Read the model definition and answer for the solid it produces. Units are mm, in the model's axes. Give positions to 0.01 mm unless a question says otherwise; leave off trailing zeros. Write each question's results on one line, items separated by ' | '.
from build123d import *

# Parameters (mm, degrees)
BOSS_EXTRUDE1_DEPTH  = 600
MIRROR3_COPY_1_DEPTH = 600
MIRROR3_COPY_2_DEPTH = 600


with BuildPart() as part:
    # Sketch1 → Boss-Extrude1 (new body)
    with BuildSketch(Plane.XY):
        with BuildLine():
            Line((3.4, 0), (5.5, 0))
            Line((5.5, 0), (5.5, 4))
            Line((5.5, 4), (11.69, 10.19))
            Line((11.69, 10.19), (18.2, 10.19))
            Line((18.2, 10.19), (18.2, 5.265595036))
            Line((18.2, 5.265595036), (15.5, 5.265595036))
            Line((15.5, 5.265595036), (15.5, 2.965595036))
            Line((15.5, 2.965595036), (19, 2.965595036))
            Line((19, 2.965595036), (19, 3.965595036))
            Line((19, 3.965595036), (20, 3.965595036))
            Line((20, 3.965595036), (20, 15.5))
            ThreePointArc((20, 15.5), (18.681980515, 18.681980515), (15.5, 20))
            Line((15.5, 20), (6.385304712, 20))
            Line((6.385304712, 20), (6.385304712, 19))
            Line((6.385304712, 19), (5.385304712, 19))
            Line((5.385304712, 19), (5.385304712, 15.5))
            Line((5.385304712, 15.5), (7.685304712, 15.5))
            Line((7.685304712, 15.5), (7.685304712, 18.2))
            Line((7.685304712, 18.2), (10.19, 18.2))
            Line((10.19, 18.2), (10.19, 11.69))
            Line((10.19, 11.69), (4, 5.5))
            Line((4, 5.5), (0, 5.5))
            Line((0, 5.5), (0, 3.4))
            ThreePointArc((0, 3.4), (2.404163056, 2.404163056), (3.4, 0))
        make_face()
        with BuildLine():
            Line((18.5, 11.69), (18.5, 15.5))
            ThreePointArc((18.5, 15.5), (17.621320344, 17.621320344), (15.5, 18.5))
            Line((15.5, 18.5), (11.69, 18.5))
            Line((11.69, 18.5), (11.69, 11.69))
            Line((11.69, 11.69), (18.5, 11.69))
        make_face(mode=Mode.SUBTRACT)
    boss_extrude1 = extrude(amount=BOSS_EXTRUDE1_DEPTH)

    # Mirror1: Boss-Extrude1 across plane
    add(boss_extrude1.mirror(Plane.ZX))

    # Mirror2: Boss-Extrude1 across plane
    add(boss_extrude1.mirror(Plane(origin=(0, 0, 0), x_dir=(0, 0, 1), z_dir=(1, 0, 0))))

    # Mirror3 copy 1 sketch → Mirror3 copy 1 (add)
    with BuildSketch(Plane(origin=(0, 0, 0), x_dir=(-1, 0, 0), z_dir=(0, 0, 1))):
        with BuildLine():
            Line((3.4, 0), (5.5, 0))
            Line((5.5, 0), (5.5, 4))
            Line((5.5, 4), (11.69, 10.19))
            Line((11.69, 10.19), (18.2, 10.19))
            Line((18.2, 10.19), (18.2, 5.265595036))
            Line((18.2, 5.265595036), (15.5, 5.265595036))
            Line((15.5, 5.265595036), (15.5, 2.965595036))
            Line((15.5, 2.965595036), (19, 2.965595036))
            Line((19, 2.965595036), (19, 3.965595036))
            Line((19, 3.965595036), (20, 3.965595036))
            Line((20, 3.965595036), (20, 15.5))
            ThreePointArc((20, 15.5), (18.681980515, 18.681980515), (15.5, 20))
            Line((15.5, 20), (6.385304712, 20))
            Line((6.385304712, 20), (6.385304712, 19))
            Line((6.385304712, 19), (5.385304712, 19))
            Line((5.385304712, 19), (5.385304712, 15.5))
            Line((5.385304712, 15.5), (7.685304712, 15.5))
            Line((7.685304712, 15.5), (7.685304712, 18.2))
            Line((7.685304712, 18.2), (10.19, 18.2))
            Line((10.19, 18.2), (10.19, 11.69))
            Line((10.19, 11.69), (4, 5.5))
            Line((4, 5.5), (0, 5.5))
            Line((0, 5.5), (0, 3.4))
            ThreePointArc((0, 3.4), (2.404163056, 2.404163056), (3.4, 0))
        make_face()
        with BuildLine():
            Line((18.5, 11.69), (18.5, 15.5))
            ThreePointArc((18.5, 15.5), (17.621320344, 17.621320344), (15.5, 18.5))
            Line((15.5, 18.5), (11.69, 18.5))
            Line((11.69, 18.5), (11.69, 11.69))
            Line((11.69, 11.69), (18.5, 11.69))
        make_face(mode=Mode.SUBTRACT)
    extrude(amount=MIRROR3_COPY_1_DEPTH)

    # Mirror3 copy 2 sketch → Mirror3 copy 2 (add)
    with BuildSketch(Plane.XY):
        with BuildLine():
            Line((3.4, 0), (5.5, 0))
            Line((5.5, 0), (5.5, -4))
            Line((5.5, -4), (11.69, -10.19))
            Line((11.69, -10.19), (18.2, -10.19))
            Line((18.2, -10.19), (18.2, -5.265595036))
            Line((18.2, -5.265595036), (15.5, -5.265595036))
            Line((15.5, -5.265595036), (15.5, -2.965595036))
            Line((15.5, -2.965595036), (19, -2.965595036))
            Line((19, -2.965595036), (19, -3.965595036))
            Line((19, -3.965595036), (20, -3.965595036))
            Line((20, -3.965595036), (20, -15.5))
            ThreePointArc((20, -15.5), (18.681980515, -18.681980515), (15.5, -20))
            Line((15.5, -20), (6.385304712, -20))
            Line((6.385304712, -20), (6.385304712, -19))
            Line((6.385304712, -19), (5.385304712, -19))
            Line((5.385304712, -19), (5.385304712, -15.5))
            Line((5.385304712, -15.5), (7.685304712, -15.5))
            Line((7.685304712, -15.5), (7.685304712, -18.2))
            Line((7.685304712, -18.2), (10.19, -18.2))
            Line((10.19, -18.2), (10.19, -11.69))
            Line((10.19, -11.69), (4, -5.5))
            Line((4, -5.5), (0, -5.5))
            Line((0, -5.5), (0, -3.4))
            ThreePointArc((0, -3.4), (2.404163056, -2.404163056), (3.4, 0))
        make_face()
        with BuildLine():
            Line((18.5, -11.69), (18.5, -15.5))
            ThreePointArc((18.5, -15.5), (17.621320344, -17.621320344), (15.5, -18.5))
            Line((15.5, -18.5), (11.69, -18.5))
            Line((11.69, -18.5), (11.69, -11.69))
            Line((11.69, -11.69), (18.5, -11.69))
        make_face(mode=Mode.SUBTRACT)
    extrude(amount=MIRROR3_COPY_2_DEPTH)


solid = part.part
(1) Consider probe 1 along X at (y, z) = (-13.5, 504); probe 2 along X at (y, z) = (4, 525). Determine where each line is inside the solid, lowest interval first. Write a range as [from, to].
Conclusion:
probe 1: [-20, -18.5], [-11.69, -10.19], [10.19, 11.69], [18.5, 20] | probe 2: [-20, -15.5], [-5.5, 5.5], [15.5, 20]
(2) Section A-A (z = 357.5) is taken. State how many separate pieces and enclosed holes the cut face has, plus the area to 3 significant figures.
Conclusion:
separate pieces: 1 | enclosed holes: 5 | area: 468 mm^2
(3) Each of these flat-tipped pins is pushed along its axis until it touches: pin 1 (1 mm diameter, centred on x = 15.5, y = -16, fed in from -Z); pin 2 (4 mm diameter, centred on y = 1, z = 181, fed in from +X); pin 3 (1.5 mm diameter, centred on x = 0.5, z = 227, fed in from -Y); pin 4 (3 mm diameter, centred on y = -17.5, z = 192.5, fed in from -X). Where does it stop, or does it pass through?
Conclusion:
pin 1: through | pin 2: x = 19 | pin 3: y = -5.5 | pin 4: x = -19.97
